from build123d import *

# Parameters (mm, degrees)
BASE_FLANGE1_DEPTH           = 170
F_30_0_1285_DIAMETER_HOLE1_D = 3.2639
FILLET1_R                    = 5


# Sheet-metal steps are written as plain solids
with BuildPart() as part:
    # Sketch1 → Base-Flange1 (new body)
    with BuildSketch(Plane.XY):
        with BuildLine():
            Line((-25.4, 0), (-6, 0))
            ThreePointArc((-6, 0), (-1.757359313, 1.757359313), (0, 6))
            Line((0, 6), (0, 50.8))
            Line((0, 50.8), (-3, 50.8))
            Line((-3, 50.8), (-3, 6))
            ThreePointArc((-3, 6), (-3.878679656, 3.878679656), (-6, 3))
            Line((-6, 3), (-25.4, 3))
            Line((-25.4, 3), (-25.4, 0))
        make_face()
    extrude(amount=BASE_FLANGE1_DEPTH)

    # #30 (0.1285) Diameter Hole1 (through all)
    with Locations(Plane(origin=(0, 3, 0), x_dir=(1, 0, 0), z_dir=(0, 1, 0))):
        with Locations((-15.7, -25), (-15.7, -75), (-15.7, -125)):
            Hole(F_30_0_1285_DIAMETER_HOLE1_D / 2)

    # Fillet1
    fillet1_edges = [part.edges().sort_by_distance(p)[0] for p in [
        (-1.5, 50.8, 170),
        (-1.5, 50.8, 0),
        (-25.4, 1.5, 170),
        (-25.4, 1.5, 0),
    ]]
    fillet(fillet1_edges, radius=FILLET1_R)


solid = part.part
Geometry: final body of the model. Coordinates: model frame, mm. A direction names the side the tool comes from. Give positions to 0.01 mm unless a question says otherwise; leave off trailing zeros. Write each loop counter-clockwise with the first axis right and the second up, starting at its lowest first coordinate (ties: lowest second). Pieces come first, ordered by that corner, then holes. Notation, with made-up numbers: (-39, 31.5) - (11, 31.5) arc R23 ccw to (11, 51.5) - close; hole circle Ø1 at (10.25, 45). An arc over 180 degrees is marked (long way). Return JSON: item names as keys, results as strings. Group by question number.
1) Mould query, pull axis X, two halves, no side actions, for faces 3 (the cylindrical face through (-15.49, 1.48, 123.38)), 4 (the flat face through (-2.7, 16.2, 170)), 5 (the flat face through (-3, 29, 84)). Classes: released by +X, released by -X, zero draft, split by the parting line, or undercut.
2) Line query: line 1 (Z direction, x = -15.7, y = 0.8); line 2 (Y direction, x = -16.5, z = 37); line 3 (X direction, y = 16, z = 42). Output: solid intervals per line, ascending.
3) Set-up query: faces 1 (the cylindrical face through (-1.52, 49.3, 168.57)), 2 (the flat face through (-16, 3, 84)). Return all of +Z, -Z, +X, -X, +Y, -Y with unobstructed straight access to the full face (end or side cutting, diameter ignored); none if empty.
4) First-contact query: P1, Ø3, axis at y = 18.5, z = 89, coming from the -X side; P2, Ø5, axis at x = -6, z = 47.5, coming from the +Y side; P3, Ø9.5, axis at x = -17.5, z = 64.5, coming from the +Y side. Flat tips, straight axial feed; report the tip coordinate or a pass-through.
5) Section B-B on z = 75. Return the cut outline in (x, y).
6) Section C-C on z = 110. Return the cut outline in (x, y).
7) Section D-D on y = 22.5. Return the cut outline in (x, z).
8) Section A-A on x = -15.7. Return the cut outline in (y, z).
Filled in:
{
 "1": {"face 3": "undercut", "face 4": "zero draft", "face 5": "released by -X"},
 "2": {"line 1": "z = 0 to 23.37, 26.63 to 73.37, 76.63 to 123.37, 126.63 to 170", "line 2": "y = 0 to 3", "line 3": "x = -3 to 0"},
 "3": {"face 1": "+Z, +X, -X, +Y", "face 2": "+Z, -Z, -X, +Y"},
 "4": {"P1": "stops at x = -3", "P2": "stops at y = 4.34", "P3": "stops at y = 3"},
 "5": {"outline": "(-25.4, 0) - (-17.33, 0) - (-17.33, 3) - (-25.4, 3) - close; (-14.07, 0) - (-6, 0) arc R6 ccw to (0, 6) - (0, 50.8) - (-3, 50.8) - (-3, 6) arc R3 cw to (-6, 3) - (-14.07, 3) - close"},
 "6": {"outline": "(-25.4, 0) - (-6, 0) arc R6 ccw to (0, 6) - (0, 50.8) - (-3, 50.8) - (-3, 6) arc R3 cw to (-6, 3) - (-25.4, 3) - close"},
 "7": {"outline": "(-3, 0) - (0, 0) - (0, 170) - (-3, 170) - close"},
 "8": {"outline": "(0, 0) - (3, 0) - (3, 23.37) - (0, 23.37) - close; (0, 26.63) - (3, 26.63) - (3, 73.37) - (0, 73.37) - close; (0, 76.63) - (3, 76.63) - (3, 123.37) - (0, 123.37) - close; (0, 126.63) - (3, 126.63) - (3, 170) - (0, 170) - close"}
}
